from build123d import *

# Parameters (mm, degrees)
BASE_EXTRUSION_DEPTH    = 12.5
CONG_1_R                = 0.5
ESQUISSE2_R             = 30
ENL_V_MAT_EXTRU_1_DEPTH = 1.5


with BuildPart() as part:
    # Esquisse1 → Base-Extrusion (new body)
    with BuildSketch(Plane.XY):
        with BuildLine():
            Line((0, -3.9), (12, -3.9))
            Line((12, -3.9), (12, -0.4))
            Line((12, -0.4), (3.879432948, -0.4))
            ThreePointArc((3.879432948, -0.4), (-2.612470096, 2.895686447), (0, -3.9))
        make_face()
    extrude(amount=BASE_EXTRUSION_DEPTH)

    # Congé1
    cong_1_edges = [part.edges().sort_by_distance(p)[0] for p in [
        (12, -3.9, 6.25),
        (12, -0.4, 6.25),
    ]]
    fillet(cong_1_edges, radius=CONG_1_R)

    # Esquisse2 → Enlèv. mat.-Extru.1 (cut)
    with BuildSketch(Plane.XY.offset(7)):
        with Locations((-15, 20)):
            Circle(ESQUISSE2_R)
    extrude(amount=-ENL_V_MAT_EXTRU_1_DEPTH, mode=Mode.SUBTRACT)


solid = part.part
The model under review builds one solid part; all positions refer to its coordinate system, in mm. A direction names the side the tool comes from. Give positions to 0.01 mm unless a question says otherwise; leave off trailing zeros. Loops run counter-clockwise (first coordinate to the right, second up) from the corner with the lowest first, then second, coordinate; pieces in that order, holes last. Notation, with made-up numbers: (-38.5, -15.5) -> (-25.5, -15.5) arc R13 cw to (-25.5, 5.5) -> close; hole circle Ø10 at (78, 52.25). An arc over 180 degrees is marked (long way). Answer as a JSON object with one key per item and string values. Group by question number.
Q1. Take a section at C-C (z = 3). Write out the cut boundary in (x, y), plus the area to 3 significant figures.
Q2. Take a section at A-A (y = 0). Write out the cut boundary in (x, z).
Q3. Tool access review of faces 5 (the cylindrical face through (-2.513, 2.982, 2.712)), 6 (the cylindrical face through (5.11, -2.26, 6.26)): name each direction out of +Z, -Z, +X, -X, +Y, -Y from which nothing blocks a thin tool from reaching the whole face with its end or side.
Q4. Wall thickness on line 1 along Z through (x, y) = (1, -1); line 2 along X through (y, z) = (0, 10.75); line 3 along Y through (x, z) = (6, 10.75): over which ranges is each line inside the solid? List them lowest first.
Q5. Insertion check: pin 1 (4 mm diameter, centred on x = 2.5, z = 5.5, fed in from +Y); pin 2 (2.5 mm diameter, centred on x = 8.5, z = 7.5, fed in from +Y). Each pin has a flat end and moves straight along its axis. Give the tip position at first contact, or say it passes through.
Q6. Draft analysis for pull direction Z (two halves, no side actions). For faces 1 (the flat face through (6, -3.9, 6)), 2 (the flat face through (0, 0, 5.5)), 3 (the flat face through (2, -1, 12.5)), 4 (the flat face through (0, 0, 7)), state which applies: pulls with the +Z half, pulls with the -Z half, needs draft (parallel to the pull), parting line crosses it, or undercut.
Q7. Take a section at D-D (y = -1.5). Write out the cut boundary in (x, z).
Q8. Take a section at B-B (x = -0.5). Write out the cut boundary in (y, z).
Answer below:
{
 "1": {"outline": "(0, -3.9) -> (11.5, -3.9) arc R0.5 ccw to (12, -3.4) -> (12, -0.9) arc R0.5 ccw to (11.5, -0.4) -> (3.88, -0.4) arc R3.9 ccw (long way) to start", "area": "79.3 mm2"},
 "2": {"outline": "(-3.9, 0) -> (3.9, 0) -> (3.9, 5.5) -> (-3.9, 5.5) -> close; (-3.9, 7) -> (3.9, 7) -> (3.9, 12.5) -> (-3.9, 12.5) -> close"},
 "3": {"face 5": "+Z, -Z", "face 6": "-X, +Y"},
 "4": {"line 1": "z = 0 to 5.5, 7 to 12.5", "line 2": "x = -3.9 to 3.9", "line 3": "y = -3.9 to -0.4"},
 "5": {"pin 1": "stops at y = 3.87", "pin 2": "stops at y = -0.4"},
 "6": {"face 1": "needs draft", "face 2": "undercut", "face 3": "pulls with the +Z half", "face 4": "undercut"},
 "7": {"outline": "(-3.6, 0) -> (12, 0) -> (12, 12.5) -> (-3.6, 12.5) -> (-3.6, 7) -> (5.92, 7) -> (5.92, 5.5) -> (-3.6, 5.5) -> close"},
 "8": {"outline": "(-3.87, 0) -> (3.87, 0) -> (3.87, 5.5) -> (-3.87, 5.5) -> close; (-3.87, 7) -> (3.87, 7) -> (3.87, 12.5) -> (-3.87, 12.5) -> close"}
}
